Source: CAD feature listing. Evaluate the final solid. Frame: model axes, mm. Coordinates: 2 decimals unless noted, no trailing zeros. Loops run counter-clockwise (first coordinate to the right, second up) from the corner with the lowest first, then second, coordinate; pieces in that order, holes last. Notation, with made-up numbers: (43, -35.5) -> (96, -35.5) arc R22 cw to (96, -2.5) -> close; hole circle Ø1 at (-31, 32). An arc over 180 degrees is marked (long way). One line per question, with ' | ' between items. Start each with the question number.
```python
from build123d import *

# Parameters (mm, degrees)
SKETCH1_R                = 5
SKETCH1_R_2              = 2
SKETCH1_R_3              = 7
SKETCH1_R_4              = 3
BOSS_EXTRUDE1_DEPTH      = 5
BOSS_EXTRUDE1_DEPTH_BACK = 5


with BuildPart() as part:
    # Sketch1 → Boss-Extrude1 (new body, two sides)
    with BuildSketch(Plane.XY) as boss_extrude1_sk:
        with BuildLine():
            Line((-228.038090057, 37.726797985), (-98.274394802, 131.307690232))
            ThreePointArc((-98.274394802, 131.307690232), (-107.99485935, 132.820161378), (-106.604012177, 142.558772375))
            Line((-106.604012177, 142.558772375), (-233.987816753, 45.76328523))
            ThreePointArc((-233.987816753, 45.76328523), (-228.740726452, 46.261375122), (-225.962721435, 41.782230305))
            ThreePointArc((-225.962721435, 41.782230305), (-226.511701502, 39.504419612), (-228.038090057, 37.726797985))
        make_face()
        with Locations((-230.962721435, 41.782230305)):
            Circle(SKETCH1_R)
        with Locations((-230.962721435, 41.782230305)):
            Circle(SKETCH1_R_2, mode=Mode.SUBTRACT)
        with Locations((-70.220418055, 160.786061774)):
            Circle(SKETCH1_R)
        with Locations((-70.220418055, 160.786061774)):
            Circle(SKETCH1_R_2, mode=Mode.SUBTRACT)
        with BuildLine():
            ThreePointArc((-95.368878731, 136.98529548), (-95.787048458, 134.602123171), (-96.991595947, 132.503685294))
            ThreePointArc((-96.991595947, 132.503685294), (-83.549961909, 145.833090362), (-67.837220551, 156.390567529))
            ThreePointArc((-67.837220551, 156.390567529), (-74.23897564, 157.810965987), (-73.728811684, 164.348529198))
            ThreePointArc((-73.728811684, 164.348529198), (-88.41310273, 152.401891111), (-105.085651055, 143.436585904))
            ThreePointArc((-105.085651055, 143.436585904), (-98.497019118, 142.816993614), (-95.368878731, 136.98529548))
        make_face()
        with Locations((-102.368878731, 136.98529548)):
            Circle(SKETCH1_R_3)
        with Locations((-102.368878731, 136.98529548)):
            Circle(SKETCH1_R_4, mode=Mode.SUBTRACT)
    extrude(amount=BOSS_EXTRUDE1_DEPTH)
    extrude(boss_extrude1_sk.sketch, amount=-BOSS_EXTRUDE1_DEPTH_BACK)


solid = part.part
```
(1) Cut plane B-B, the plane x = -150. Return the cut outline in (y, z).
(2) Cut plane C-C, the plane y = 64. Return the cut outline in (x, z), and give its area (3 significant figures).
(3) Ray query, L1, parallel to X at y = 102, z = -1; L2, parallel to X at y = 142.5, z = -3.75; L3, parallel to Y at x = -218, z = -4.25. Return the intervals inside material, ascending.
(4) Cut plane A-A, the plane z = 2.5. Return the cut outline in (x, y).
(5) Contact query for flat-ended pins moving along their axis: pin 1 Ø9.5 at (x, y) = (-102.37, 136.99) entering from -Z; pin 2 Ø2 at (y, z) = (141.5, -3.5) entering from +X; pin 3 Ø3 at (x, y) = (-70.22, 160.79) entering from -Z; pin 4 Ø5 at (y, z) = (100.5, 2.5) entering from +X. Output: stop coordinate, or through.
(6) Draft query along Y for faces 1 (the cylindrical face through (-232.96, 41.87, -0.07)), 2 (the cylindrical face through (-69.3, 159.01, -0.07)), 3 (the cylindrical face through (-88.19, 152.55, 0.07)), 4 (the flat face through (-164.065, 83.862, 0.07)). Return one class per face: pulls with the +Y half, pulls with the -Y half, needs draft (parallel to the pull), parting line crosses it, or undercut.
Here are the results:
1) outline: (94.01, -5) -> (109.58, -5) -> (109.58, 5) -> (94.01, 5) -> close
2) outline: (-209.99, -5) -> (-191.61, -5) -> (-191.61, 5) -> (-209.99, 5) -> close | area: 184 mm2
3) L1: x = -159.98 to -138.91 | L2: x = -106.68 to -87.41 | L3: y = 44.97 to 57.91
4) outline: (-233.99, 45.76) arc R5 ccw to (-228.04, 37.73) -> (-98.27, 131.31) arc R7 ccw to (-96.99, 132.5) arc R100 cw to (-67.84, 156.39) arc R5 ccw (long way) to (-73.73, 164.35) arc R100 cw to (-105.09, 143.44) arc R7 ccw to (-106.6, 142.56) -> close; hole circle Ø4 at (-230.96, 41.78); hole circle Ø6 at (-102.37, 136.99); hole circle Ø4 at (-70.22, 160.79)
5) pin 1: stops at z = -5 | pin 2: stops at x = -87.41 | pin 3: passes through | pin 4: stops at x = -137.53
6) face 1: undercut | face 2: undercut | face 3: pulls with the +Y half | face 4: pulls with the -Y half
